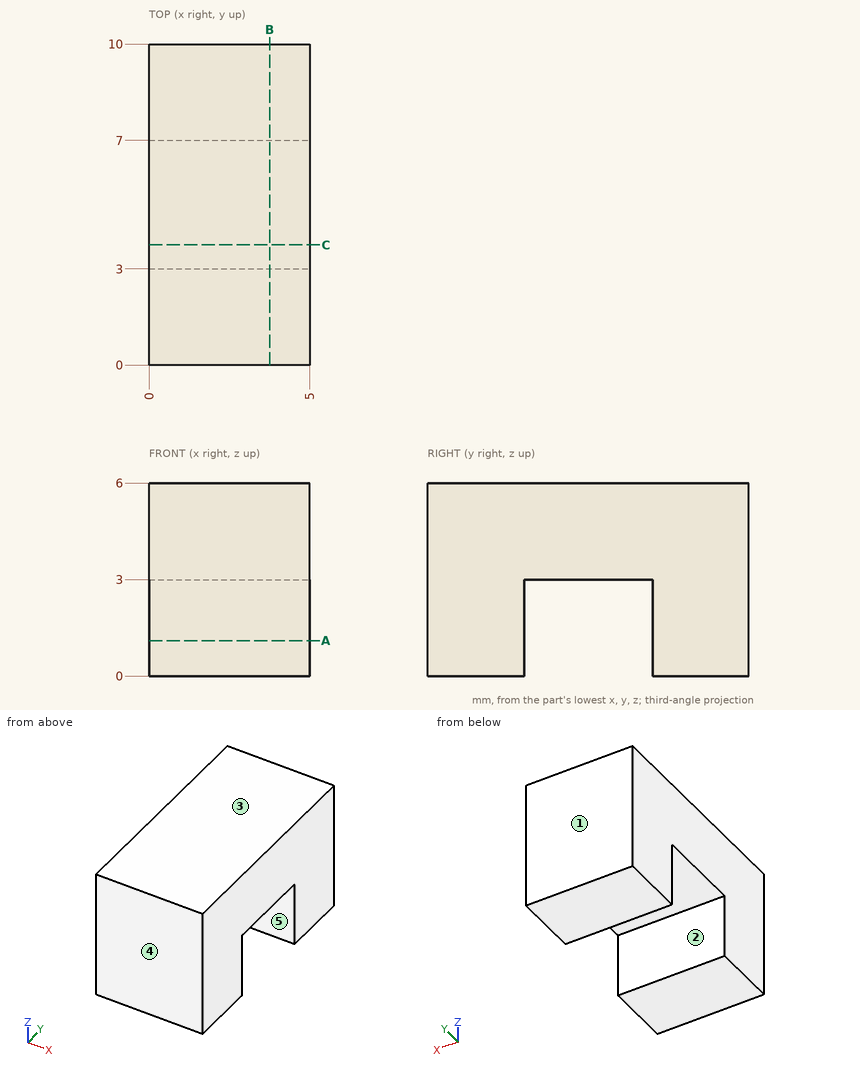
Design review of the part shown in the three views and the two pictorial views. Dimensions are in mm from the part's minimum x, y and z. A direction names the side the tool comes from. Coordinates: 2 decimals unless noted, no trailing zeros. Write each loop counter-clockwise with the first axis right and the second up, starting at its lowest first coordinate (ties: lowest second). Pieces come first, ordered by that corner, then holes.
1) We need section C-C on y = 3.75. State the section outline as (x, z) points, then the cut area to 3 significant figures.
2) We need section A-A on z = 1.1. State the section outline as (x, y) points, then the cut area to 3 significant figures.
3) To check wall thickness, follow probe 1 along Y at (x, z) = (2.1, 1.9); probe 2 along Z at (x, y) = (2.25, 4.75). State the ranges of each line that lie inside material, in increasing order.
4) We need section B-B on x = 3.75. State the section outline as (y, z) points, then the cut area to 3 significant figures.
5) Machinability: for the marked faces 1 and 2, which of the approach directions +Z, -Z, +X, -X, +Y, -Y give a long, thin tool a straight path to every point of the face, cutting with its end or side? Answer none if there is none.
6) The part is to be moulded in two halves that separate along Y. For the marked faces 3, 4 and 5, say which applies: pulls with the +Y half, pulls with the -Y half, needs draft (parallel to the pull), parting line crosses it, or undercut.
7) Clearance check with a flat-ended pin moving along its axis: pin 1 Ø2 at (x, y) = (1.5, 4.5) entering from -Z. State where the tip first meets the part, or that it passes through.
Answer list:
1. outline: (0, 3) - (5, 3) - (5, 6) - (0, 6) - close
1. area: 15.0 mm2
2. outline: (0, 0) - (5, 0) - (5, 3) - (0, 3) - close; (0, 7) - (5, 7) - (5, 10) - (0, 10) - close
2. area: 30.0 mm2
3. probe 1: y = 0 to 3, 7 to 10
3. probe 2: z = 3 to 6
4. outline: (0, 0) - (3, 0) - (3, 3) - (7, 3) - (7, 0) - (10, 0) - (10, 6) - (0, 6) - close
4. area: 48.0 mm2
5. face 1: +Z, -Z, +X, -X, +Y
5. face 2: -Z, +X, -X
6. face 3: needs draft
6. face 4: pulls with the -Y half
6. face 5: undercut
7. pin 1: stops at z = 3
